For this review, use the dimensioned drawing (mm, ordinates from the lowest corner) and the shaded views. Give positions to 0.01 mm unless a question says otherwise; leave off trailing zeros. Order: outer loops, then holes, each group sorted by start corner. A loop starts at its lowest first (then second) coordinate and runs counter-clockwise, first axis right, second up.
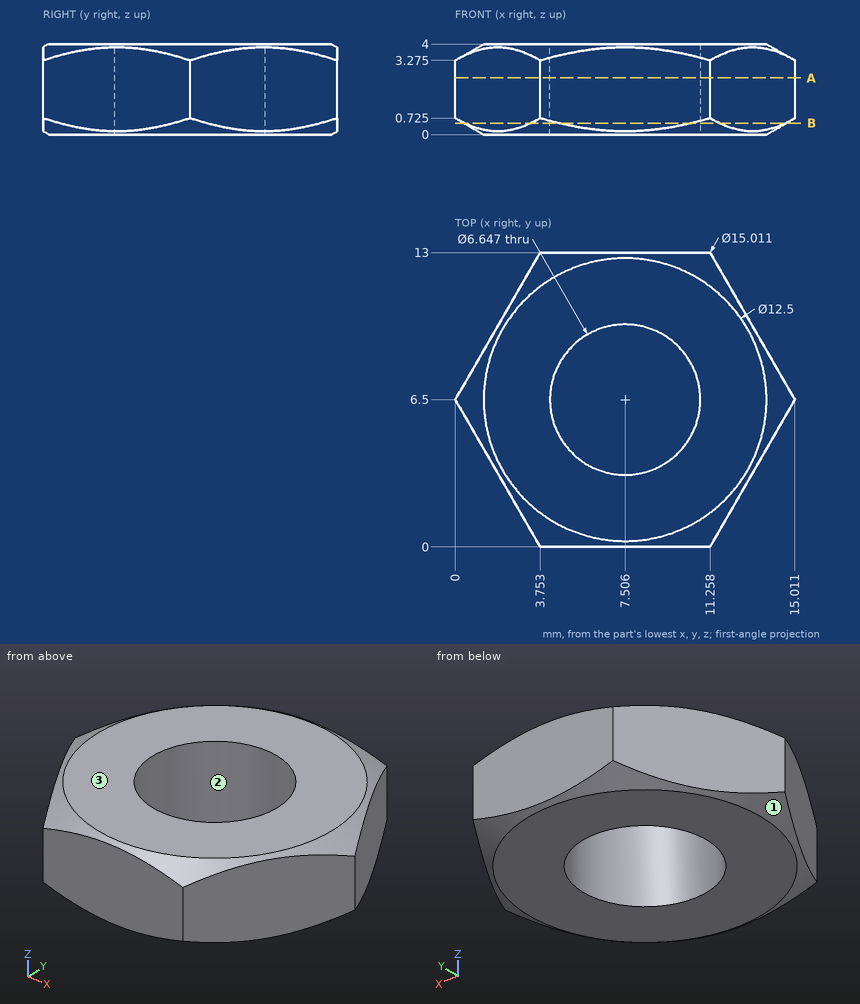
1. Draft analysis for pull direction Y (two halves, no side actions). For the marked faces 1, 2 and 3, state which applies: pulls with the +Y half, pulls with the -Y half, needs draft (parallel to the pull), parting line crosses it, or undercut.
Recorded:
face 1: parting line crosses it
face 2: undercut
face 3: needs draft
2. Take a section at B-B (z = 0.5). State the section outline as (x, y) points (1 decimal), then the cut area to 3 significant figures.
Recorded:
outline: (0.4, 5.8) - (3.3, 0.7) arc R7.1 ccw to (4.6, 0) - (10.4, 0) arc R7.1 ccw to (11.7, 0.7) - (14.6, 5.8) arc R7.1 ccw to (14.6, 7.2) - (11.7, 12.3) arc R7.1 ccw to (10.4, 13) - (4.6, 13) arc R7.1 ccw to (3.3, 12.3) - (0.4, 7.2) arc R7.1 ccw to start; hole circle Ø6.6 at (7.5, 6.5)
area: 110 mm2
3. For pin 1 (1 mm diameter, centred on y = 3, z = 1.5, fed in from +X), flat-tipped, find the tip position at first contact; note if it passes through.
Recorded:
pin 1: stops at x = 13.28
4. For line 1 along Y through (x, z) = (7.5, 1.9); line 2 along X through (y, z) = (8.25, 3.85) (1 decimal); line 3 along Y through (x, z) = (9.75, 1.35), list the stretches that pass through material, from the lowest coordinate up.
Recorded:
line 1: y = 0 to 3.18, 9.82 to 13
line 2: x = 1.2 to 4.7, 10.3 to 13.8
line 3: y = 0 to 4.05, 8.95 to 13
5. Take a section at A-A (z = 2.5). State the section outline as (x, y) points (1 decimal).
Recorded:
outline: (0, 6.5) - (3.8, 0) - (11.3, 0) - (15, 6.5) - (11.3, 13) - (3.8, 13) - close; hole circle Ø6.6 at (7.5, 6.5)
